```python
from build123d import *


with BuildPart() as part:
    # BodySke → Body (revolve)
    with BuildSketch(Plane.XY, mode=Mode.PRIVATE) as body_sk:
        with BuildLine():
            Line((2, 8), (73, 8.709999999))
            Line((73, 8.709999999), (75, 8.174101614))
            Line((75, 8.174101614), (75, 5.25))
            Line((75, 5.25), (73.5, 5.25))
            Line((73.5, 5.25), (72.922649731, 4.25))
            Line((72.922649731, 4.25), (50, 4.25))
            Line((50, 4.25), (48.23959236, 0))
            Line((48.23959236, 0), (0, 0))
            ThreePointArc((0, 0), (0.507577498, 4.123105626), (2, 8))
        make_face()
    revolve(body_sk.sketch.rotate(Axis((0, 0, 0), (1, 0, 0)), 90), axis=Axis((0, 0, 0), (1, 0, 0)))


solid = part.part
```
Can you work these out from the model? Positions are in its coordinate system, mm. Round coordinates to 2 decimals unless told otherwise and drop trailing zeros. Loops run counter-clockwise (first coordinate to the right, second up) from the corner with the lowest first, then second, coordinate; pieces in that order, holes last.
Item 1: Please list where these lines run through material, in increasing order: L1, parallel to Y at x = 59.25, z = 0; L2, parallel to Y at x = 74.15, z = 0; L3, parallel to X at y = -2.5, z = 0.75.
Item 2: Suppose I cut it at A-A, the plane x = 17. Write out the boundary of the cut face in (y, z).
Item 3: If we mould it in two halves opening along Z, with no side actions, what happens to faces 1 (the flat face through (75, 5.3, 1.7)), 2 (the cylindrical face through (61.301, -4.214, -0.553)), 3 (the conical face through (38, 8.16, -1.81))? For each: +Z half, -Z half, draft (parallel to the pull), parting line (faces both ways), or undercut.
Item 4: Will these pins go through, and if not, where does the flat tip stop? pin 1 Ø4 at (x, z) = (22, -5.5) entering from +Y; pin 2 Ø4 at (x, y) = (55, -2.5) entering from +Z; pin 3 Ø1 at (x, y) = (36.5, 5.5) entering from -Z.
Reported:
1. L1: y = -8.57 to -4.25, 4.25 to 8.57
1. L2: y = -8.4 to -5.25, 5.25 to 8.4
1. L3: x = 0.2 to 49.32
2. outline: circle Ø16.3 at (0, 0)
3. face 1: draft
3. face 2: undercut
3. face 3: parting line
4. pin 1: stops at y = 7.42
4. pin 2: stops at z = 8.52
4. pin 3: stops at z = -6.68
